from build123d import *

# Parameters (mm, degrees)
F1_W     = 30
F1_H     = 15
F1_W_2   = 12.75
F1_H_2   = 5
F1_W_3   = 20
F1_W_4   = 74.5
F1_H_3   = 12.5
F1_H_4   = 8.75
F3_DEPTH = 5
F2_W     = 18.4
F2_H     = 69
F4_DEPTH = 5


with BuildPart() as f3:
    # F1 (on Top) → F3 (new body)
    with BuildSketch(Plane.XY):
        with BuildLine():
            Line((50, 100), (-50, 100))
            Line((-50, 100), (-50, 50))
            Line((-50, 50), (-37.25, 50))
            Line((-37.25, 50), (-37.25, 70.75))
            ThreePointArc((-37.25, 70.75), (-38.4874368671, 73.7374368671), (-35.5, 72.5))
            Line((-35.5, 72.5), (35.5, 72.5))
            ThreePointArc((35.5, 72.5), (37.25, 74.25), (39, 72.5))
            ThreePointArc((39, 72.5), (38.4874368671, 71.2625631329), (37.25, 70.75))
            Line((37.25, 70.75), (37.25, 50))
            Line((37.25, 50), (50, 50))
            Line((50, 50), (50, 100))
        make_face()
        with Locations((-30, 87.5)):
            Rectangle(F1_W, F1_H, mode=Mode.SUBTRACT)
        with Locations((30, 87.5)):
            Rectangle(F1_W, F1_H, mode=Mode.SUBTRACT)
        with Locations((-43.625, 47.5)):
            Rectangle(F1_W_2, F1_H_2)
        with BuildLine():
            Line((-50, 45), (-50, 50))
            Line((-50, 50), (-75, 50))
            Line((-75, 50), (-75, -50))
            Line((-75, -50), (-50, -50))
            Line((-50, -50), (-50, -45))
            Line((-50, -45), (-70, -45))
            Line((-70, -45), (-70, -15))
            Line((-70, -15), (-50, -15))
            Line((-50, -15), (-50, -6.25))
            Line((-50, -6.25), (-65.75, -6.25))
            ThreePointArc((-65.75, -6.25), (-68.7374368671, -7.4874368671), (-67.5, -4.5))
            Line((-67.5, -4.5), (-67.5, 4.5))
            ThreePointArc((-67.5, 4.5), (-68.7374368671, 7.4874368671), (-65.75, 6.25))
            Line((-65.75, 6.25), (-50, 6.25))
            Line((-50, 6.25), (-50, 15))
            Line((-50, 15), (-70, 15))
            Line((-70, 15), (-70, 45))
            Line((-70, 45), (-50, 45))
        make_face()
        with BuildLine():
            Line((75, 50), (50, 50))
            Line((50, 50), (50, 45))
            Line((50, 45), (70, 45))
            Line((70, 45), (70, 15))
            Line((70, 15), (50, 15))
            Line((50, 15), (50, 6.25))
            Line((50, 6.25), (65.75, 6.25))
            ThreePointArc((65.75, 6.25), (67.5, 8), (69.25, 6.25))
            ThreePointArc((69.25, 6.25), (68.7374368671, 5.0125631329), (67.5, 4.5))
            Line((67.5, 4.5), (67.5, -4.5))
            ThreePointArc((67.5, -4.5), (68.7374368671, -5.0125631329), (69.25, -6.25))
            ThreePointArc((69.25, -6.25), (67.5, -8), (65.75, -6.25))
            Line((65.75, -6.25), (50, -6.25))
            Line((50, -6.25), (50, -15))
            Line((50, -15), (70, -15))
            Line((70, -15), (70, -45))
            Line((70, -45), (50, -45))
            Line((50, -45), (50, -50))
            Line((50, -50), (75, -50))
            Line((75, -50), (75, 50))
        make_face()
        with Locations((43.625, 47.5)):
            Rectangle(F1_W_2, F1_H_2)
        with BuildLine():
            Line((-37.25, -50), (-50, -50))
            Line((-50, -50), (-50, -100))
            Line((-50, -100), (50, -100))
            Line((50, -100), (50, -50))
            Line((50, -50), (37.25, -50))
            Line((37.25, -50), (37.25, -70.75))
            ThreePointArc((37.25, -70.75), (38.4874368671, -71.2625631329), (39, -72.5))
            ThreePointArc((39, -72.5), (37.25, -74.25), (35.5, -72.5))
            Line((35.5, -72.5), (-35.5, -72.5))
            ThreePointArc((-35.5, -72.5), (-38.4874368671, -73.7374368671), (-37.25, -70.75))
            Line((-37.25, -70.75), (-37.25, -50))
        make_face()
        with Locations((-35, -87.5)):
            Rectangle(F1_W_3, F1_H, mode=Mode.SUBTRACT)
        with Locations((35, -87.5)):
            Rectangle(F1_W_3, F1_H, mode=Mode.SUBTRACT)
        with Locations((-43.625, -47.5)):
            Rectangle(F1_W_2, F1_H_2)
        with Locations((43.625, -47.5)):
            Rectangle(F1_W_2, F1_H_2)
        with BuildLine():
            Line((37.25, -50), (-37.25, -50))
            Line((-37.25, -50), (-37.25, -70.75))
            ThreePointArc((-37.25, -70.75), (-36.0125631329, -71.2625631329), (-35.5, -72.5))
            Line((-35.5, -72.5), (35.5, -72.5))
            ThreePointArc((35.5, -72.5), (36.0125631329, -71.2625631329), (37.25, -70.75))
            Line((37.25, -70.75), (37.25, -50))
        make_face()
        Polygon((-37.25, -45), (-37.25, -50), (37.25, -50), (37.25, -45), (25, -45), (25, -15), (37.25, -15), (37.25, -6.25), (-37.25, -6.25), (-37.25, -15), (-25, -15), (-25, -45), align=None)
        Polygon((37.25, 50), (-37.25, 50), (-37.25, 45), (-25, 45), (-25, 15), (-37.25, 15), (-37.25, 6.25), (37.25, 6.25), (37.25, 15), (25, 15), (25, 45), (37.25, 45), align=None)
        with BuildLine():
            Line((-37.25, 70.75), (-37.25, 50))
            Line((-37.25, 50), (37.25, 50))
            Line((37.25, 50), (37.25, 70.75))
            ThreePointArc((37.25, 70.75), (36.0125631329, 71.2625631329), (35.5, 72.5))
            Line((35.5, 72.5), (-35.5, 72.5))
            ThreePointArc((-35.5, 72.5), (-36.0125631329, 71.2625631329), (-37.25, 70.75))
        make_face()
        Rectangle(F1_W_4, F1_H_3)
        with Locations((-43.625, 10.625)):
            Rectangle(F1_W_2, F1_H_4)
        with Locations((-43.625, -10.625)):
            Rectangle(F1_W_2, F1_H_4)
        with Locations((-43.625, 0)):
            Rectangle(F1_W_2, F1_H_3)
        with Locations((43.625, -10.625)):
            Rectangle(F1_W_2, F1_H_4)
        with Locations((43.625, 0)):
            Rectangle(F1_W_2, F1_H_3)
        with Locations((43.625, 10.625)):
            Rectangle(F1_W_2, F1_H_4)
        with BuildLine():
            Line((65.75, 6.25), (50, 6.25))
            Line((50, 6.25), (50, -6.25))
            Line((50, -6.25), (65.75, -6.25))
            ThreePointArc((65.75, -6.25), (66.2625631329, -5.0125631329), (67.5, -4.5))
            Line((67.5, -4.5), (67.5, 4.5))
            ThreePointArc((67.5, 4.5), (66.2625631329, 5.0125631329), (65.75, 6.25))
        make_face()
        with BuildLine():
            Line((-50, -6.25), (-50, 6.25))
            Line((-50, 6.25), (-65.75, 6.25))
            ThreePointArc((-65.75, 6.25), (-66.2625631329, 5.0125631329), (-67.5, 4.5))
            Line((-67.5, 4.5), (-67.5, -4.5))
            ThreePointArc((-67.5, -4.5), (-66.2625631329, -5.0125631329), (-65.75, -6.25))
            Line((-65.75, -6.25), (-50, -6.25))
        make_face()
    extrude(amount=F3_DEPTH)

    # F2 (on face) → F4 (cut)
    with BuildSketch(Plane.XY):
        with BuildLine():
            Line((15.25, -85), (14, -85))
            ThreePointArc((14, -85), (15.25, -86.25), (16.5, -85))
            ThreePointArc((16.5, -85), (16.1338834765, -84.1161165235), (15.25, -83.75))
            Line((15.25, -83.75), (15.25, -85))
        make_face()
        with BuildLine():
            ThreePointArc((-1.25, -85), (-0.8838834765, -85.8838834765), (0, -86.25))
            Line((0, -86.25), (0, -85))
            Line((0, -85), (-1.25, -85))
        make_face()
        with BuildLine():
            Line((0, -83.75), (0, -85))
            Line((0, -85), (1.25, -85))
            ThreePointArc((1.25, -85), (0.8838834765, -84.1161165235), (0, -83.75))
        make_face()
        with BuildLine():
            Line((0, -85), (0, -86.25))
            ThreePointArc((0, -86.25), (0.8838834765, -85.8838834765), (1.25, -85))
            Line((1.25, -85), (0, -85))
        make_face()
        with BuildLine():
            Line((-1.25, -85), (0, -85))
            Line((0, -85), (0, -83.75))
            ThreePointArc((0, -83.75), (-0.8838834765, -84.1161165235), (-1.25, -85))
        make_face()
        with BuildLine():
            ThreePointArc((0, -93.75), (-1.25, -95), (0, -96.25))
            Line((0, -96.25), (0, -93.75))
        make_face()
        with BuildLine():
            Line((0, -93.75), (0, -96.25))
            ThreePointArc((0, -96.25), (0.8838834765, -95.8838834765), (1.25, -95))
            ThreePointArc((1.25, -95), (0.8838834765, -94.1161165235), (0, -93.75))
        make_face()
        with BuildLine():
            ThreePointArc((15.25, -83.75), (14.3661165235, -84.1161165235), (14, -85))
            Line((14, -85), (15.25, -85))
            Line((15.25, -85), (15.25, -83.75))
        make_face()
        with BuildLine():
            ThreePointArc((-15.25, -83.75), (-16.1338834765, -85.8838834765), (-14, -85))
            Line((-14, -85), (-15.25, -85))
            Line((-15.25, -85), (-15.25, -83.75))
        make_face()
        with BuildLine():
            Line((-15.25, -85), (-14, -85))
            ThreePointArc((-14, -85), (-14.3661165235, -84.1161165235), (-15.25, -83.75))
            Line((-15.25, -83.75), (-15.25, -85))
        make_face()
        with BuildLine():
            Line((15.25, -54.5), (15.25, -55.75))
            ThreePointArc((15.25, -55.75), (16.1338834765, -55.3838834765), (16.5, -54.5))
            ThreePointArc((16.5, -54.5), (15.25, -53.25), (14, -54.5))
            Line((14, -54.5), (15.25, -54.5))
        make_face()
        with BuildLine():
            ThreePointArc((14, -54.5), (14.3661165235, -55.3838834765), (15.25, -55.75))
            Line((15.25, -55.75), (15.25, -54.5))
            Line((15.25, -54.5), (14, -54.5))
        make_face()
        with BuildLine():
            Line((-15.25, -54.5), (-15.25, -55.75))
            ThreePointArc((-15.25, -55.75), (-14.3661165235, -55.3838834765), (-14, -54.5))
            Line((-14, -54.5), (-15.25, -54.5))
        make_face()
        with BuildLine():
            ThreePointArc((-14, -54.5), (-16.1338834765, -53.6161165235), (-15.25, -55.75))
            Line((-15.25, -55.75), (-15.25, -54.5))
            Line((-15.25, -54.5), (-14, -54.5))
        make_face()
        with BuildLine():
            Line((17.2, -42.5), (15.95, -42.5))
            ThreePointArc((15.95, -42.5), (17.2, -43.75), (18.45, -42.5))
            ThreePointArc((18.45, -42.5), (18.0838834765, -41.6161165235), (17.2, -41.25))
            Line((17.2, -41.25), (17.2, -42.5))
        make_face()
        with BuildLine():
            ThreePointArc((17.2, -41.25), (16.3161165235, -41.6161165235), (15.95, -42.5))
            Line((15.95, -42.5), (17.2, -42.5))
            Line((17.2, -42.5), (17.2, -41.25))
        make_face()
        with BuildLine():
            Line((-17.2, -42.5), (-15.95, -42.5))
            ThreePointArc((-15.95, -42.5), (-16.3161165235, -41.6161165235), (-17.2, -41.25))
            Line((-17.2, -41.25), (-17.2, -42.5))
        make_face()
        with BuildLine():
            ThreePointArc((-17.2, -41.25), (-18.0838834765, -43.3838834765), (-15.95, -42.5))
            Line((-15.95, -42.5), (-17.2, -42.5))
            Line((-17.2, -42.5), (-17.2, -41.25))
        make_face()
        with BuildLine():
            ThreePointArc((-15.95, 42.5), (-18.0838834765, 43.3838834765), (-17.2, 41.25))
            Line((-17.2, 41.25), (-17.2, 42.5))
            Line((-17.2, 42.5), (-15.95, 42.5))
        make_face()
        with BuildLine():
            Line((-17.2, 42.5), (-17.2, 41.25))
            ThreePointArc((-17.2, 41.25), (-16.3161165235, 41.6161165235), (-15.95, 42.5))
            Line((-15.95, 42.5), (-17.2, 42.5))
        make_face()
        with BuildLine():
            ThreePointArc((15.95, 42.5), (16.3161165235, 41.6161165235), (17.2, 41.25))
            Line((17.2, 41.25), (17.2, 42.5))
            Line((17.2, 42.5), (15.95, 42.5))
        make_face()
        with BuildLine():
            Line((17.2, 42.5), (17.2, 41.25))
            ThreePointArc((17.2, 41.25), (18.0838834765, 41.6161165235), (18.45, 42.5))
            ThreePointArc((18.45, 42.5), (17.2, 43.75), (15.95, 42.5))
            Line((15.95, 42.5), (17.2, 42.5))
        make_face()
        Rectangle(F2_W, F2_H)
    extrude(amount=F4_DEPTH, mode=Mode.SUBTRACT)


solid = f3.part
Check sheet for the modelled part. Datum: model origin and axes. Units: mm. A direction names the side the tool comes from. Coordinates: 2 decimals unless noted, no trailing zeros. Write each loop counter-clockwise with the first axis right and the second up, starting at its lowest first coordinate (ties: lowest second). Pieces come first, ordered by that corner, then holes.
Item 1: Cross-section at A-A on x = 53. Record the boundary of the cut face in (y, z).
Numbers:
outline: (-50, 0) - (-45, 0) - (-45, 5) - (-50, 5) - close; (-15, 0) - (15, 0) - (15, 5) - (-15, 5) - close; (45, 0) - (50, 0) - (50, 5) - (45, 5) - close
Item 2: Mould release check, pull along X, two halves, no side actions. Record for faces 4 (the face through (-63, -50, 2)), 5 (the face through (75, -1, 2)), 6 (the face through (-47, 15, 2)), 7 (the face through (25, -30, 2)): released by +X, released by -X, zero draft, split by the parting line, or undercut.
Numbers:
face 4: zero draft
face 5: released by +X
face 6: undercut
face 7: undercut
Item 3: Scan lines: probe 1 along Y at (x, z) = (-17.2, 1.45); probe 2 along Y at (x, z) = (-60.5, 3.65); probe 3 along Y at (x, z) = (-15.25, 3.2). Record each from-to range of solid material in increasing order.
Numbers:
probe 1: y = -100 to -43.75, -41.25 to 41.25, 43.75 to 80, 95 to 100
probe 2: y = -50 to -45, -15 to 15, 45 to 50
probe 3: y = -100 to -86.25, -83.75 to -55.75, -53.25 to 80, 95 to 100
Item 4: Cross-section at C-C on z = 4.1. Count the separate pieces of the cut face and the enclosed holes in it, then the cut area to 3 significant figures.
Numbers:
separate pieces: 1
enclosed holes: 27
area: 16,700 mm2
Item 5: Access from +Z, -Z, +X, -X, +Y, -Y to the whole of each face (thin tool, end or side, straight path). Record for faces 1 (the face through (-62, 50, 2)), 2 (the face through (-25, -30, 2)), 3 (the face through (50, 75, 2)).
Numbers:
face 1: +Z, -Z, -X, +Y
face 2: +Z, -Z
face 3: +Z, -Z, +X, +Y
Item 6: Cross-section at B-B on y = 18.5. Record the boundary of the cut face in (x, z).
Numbers:
outline: (-75, 0) - (-70, 0) - (-70, 5) - (-75, 5) - close; (-25, 0) - (-9.2, 0) - (-9.2, 5) - (-25, 5) - close; (9.2, 0) - (25, 0) - (25, 5) - (9.2, 5) - close; (70, 0) - (75, 0) - (75, 5) - (70, 5) - close
Item 7: Depth check by flat-ended pin: pin 1 Ø5.5 at (x, y) = (-67.5, 6.25) entering from -Z; pin 2 Ø2 at (x, y) = (-37.25, 72.5) entering from -Z; pin 3 Ø2.5 at (y, z) = (-63.5, 1.5) entering from -X; pin 4 Ø2.5 at (x, z) = (-57, 1.5) entering from -Y. Enter the tip coordinate at first touch or a pass-through.
Numbers:
pin 1: stops at z = 0
pin 2: passes through
pin 3: stops at x = -50
pin 4: stops at y = -50
